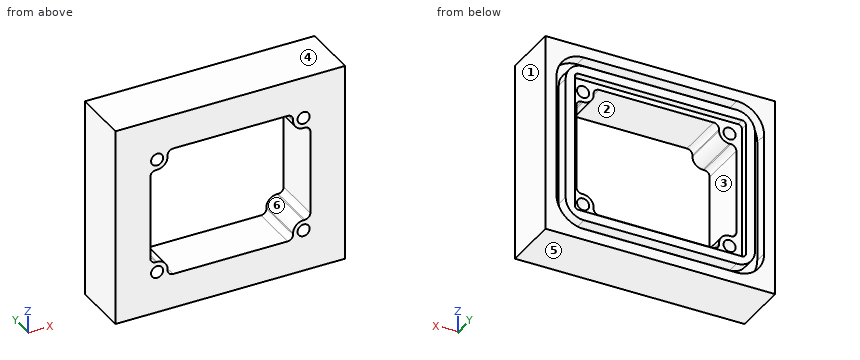
```python
from build123d import *

# Parameters (mm, degrees)
SKETCH1_W           = 62.705
SKETCH1_H           = 54.455
SKETCH1_R           = 1.65288
BOSS_EXTRUDE1_DEPTH = 15.5
SKETCH2_W           = 46.705
SKETCH2_H           = 38.455
CUT_EXTRUDE1_DEPTH  = 2.024
FILLET2_R           = 1.5
SKETCH3_W           = 56.705
SKETCH3_H           = 48.455
SKETCH3_W_2         = 51.705
SKETCH3_H_2         = 43.455
CUT_EXTRUDE2_DEPTH  = 3.5
FILLET3_R           = 1
FILLET4_R           = 5
FILLET5_R           = 7.5


with BuildPart() as part:
    # Sketch1 → Boss-Extrude1 (new body)
    with BuildSketch(Plane(origin=(0, 0, 0), x_dir=(1, 0, 0), z_dir=(0, 1, 0))):
        Rectangle(SKETCH1_W, SKETCH1_H)
        with Locations(Location((-19.995, 15.87, 0), (0, 0, 270))):
            Circle(SKETCH1_R, mode=Mode.SUBTRACT)
        with Locations(Location((19.995, 15.87, 0), (0, 0, 90))):
            Circle(SKETCH1_R, mode=Mode.SUBTRACT)
        with Locations(Location((19.995, -15.87, 0), (0, 0, 270))):
            Circle(SKETCH1_R, mode=Mode.SUBTRACT)
        with Locations(Location((-19.995, -15.87, 0), (0, 0, 90))):
            Circle(SKETCH1_R, mode=Mode.SUBTRACT)
        with BuildLine():
            Line((21.8525, 13.0125), (21.8525, -13.0125))
            Line((21.8525, -13.0125), (19.995, -13.0125))
            ThreePointArc((19.995, -13.0125), (17.974442373, -13.849442373), (17.1375, -15.87))
            Line((17.1375, -15.87), (17.1375, -17.7275))
            Line((17.1375, -17.7275), (-17.1375, -17.7275))
            Line((-17.1375, -17.7275), (-17.1375, -15.87))
            ThreePointArc((-17.1375, -15.87), (-17.974442373, -13.849442373), (-19.995, -13.0125))
            Line((-19.995, -13.0125), (-21.8525, -13.0125))
            Line((-21.8525, -13.0125), (-21.8525, 13.0125))
            Line((-21.8525, 13.0125), (-19.995, 13.0125))
            ThreePointArc((-19.995, 13.0125), (-17.974442373, 13.849442373), (-17.1375, 15.87))
            Line((-17.1375, 15.87), (-17.1375, 17.7275))
            Line((-17.1375, 17.7275), (17.1375, 17.7275))
            Line((17.1375, 17.7275), (17.1375, 15.87))
            ThreePointArc((17.1375, 15.87), (17.974442373, 13.849442373), (19.995, 13.0125))
            Line((19.995, 13.0125), (21.8525, 13.0125))
        make_face(mode=Mode.SUBTRACT)
    extrude(amount=BOSS_EXTRUDE1_DEPTH)

    # Sketch2 → Cut-Extrude1 (cut)
    with BuildSketch(Plane(origin=(0, 15.5, 0), x_dir=(1, 0, 0), z_dir=(0, 1, 0))):
        Rectangle(SKETCH2_W, SKETCH2_H)
    extrude(amount=-CUT_EXTRUDE1_DEPTH, mode=Mode.SUBTRACT)

    # Fillet2
    fillet2_edges = [part.edges().sort_by_distance(p)[0] for p in [
        (21.8525, 6.738, -13.0125),
        (21.8525, 6.738, 13.0125),
        (17.1375, 6.738, 17.7275),
        (-17.1375, 6.738, 17.7275),
        (-21.8525, 6.738, 13.0125),
        (-21.8525, 6.738, -13.0125),
        (-17.1375, 6.738, -17.7275),
        (17.1375, 6.738, -17.7275),
    ]]
    fillet(fillet2_edges, radius=FILLET2_R)

    # Sketch3 → Cut-Extrude2 (cut)
    with BuildSketch(Plane(origin=(0, 15.5, 0), x_dir=(1, 0, 0), z_dir=(0, 1, 0))):
        Rectangle(SKETCH3_W, SKETCH3_H)
        Rectangle(SKETCH3_W_2, SKETCH3_H_2, mode=Mode.SUBTRACT)
    extrude(amount=-CUT_EXTRUDE2_DEPTH, mode=Mode.SUBTRACT)

    # Fillet3
    fillet3_edges = [part.edges().sort_by_distance(p)[0] for p in [
        (-23.3525, 14.488, 19.2275),
        (-23.3525, 14.488, -19.2275),
        (23.3525, 14.488, -19.2275),
        (23.3525, 14.488, 19.2275),
    ]]
    fillet(fillet3_edges, radius=FILLET3_R)

    # Fillet4
    fillet4_edges = [part.edges().sort_by_distance(p)[0] for p in [
        (-25.8525, 13.75, 21.7275),
        (-25.8525, 13.75, -21.7275),
        (25.8525, 13.75, -21.7275),
        (25.8525, 13.75, 21.7275),
    ]]
    fillet(fillet4_edges, radius=FILLET4_R)

    # Fillet5
    fillet5_edges = [part.edges().sort_by_distance(p)[0] for p in [
        (-28.3525, 13.75, 24.2275),
        (-28.3525, 13.75, -24.2275),
        (28.3525, 13.75, -24.2275),
        (28.3525, 13.75, 24.2275),
    ]]
    fillet(fillet5_edges, radius=FILLET5_R)


solid = part.part
```
Verification items for the finished model (mm, model axes). Face numbers are marked on the shaded views. A direction names the side the tool comes from. Coordinates: 2 decimals unless noted, no trailing zeros. Loops run counter-clockwise (first coordinate to the right, second up) from the corner with the lowest first, then second, coordinate; pieces in that order, holes last. Notation, with made-up numbers: (-9, 68.5) - (29, 68.5) arc R17 cw to (29, 77.5) - close; hole circle Ø9 at (23, -16.75). An arc over 180 degrees is marked (long way). Put each result on its own line as item: value.
Item 1: Set-up check for the marked faces 5 and 6: record each of +Z, -Z, +X, -X, +Y, -Y from which the full face is reachable in a straight line by a thin tool's end or side.
Conclusion:
face 5: -Z, +X, -X, +Y, -Y
face 6: +Y, -Y
Item 2: Scan lines: line 1 along X through (y, z) = (4.25, 15.87); line 2 along Z through (x, y) = (-2.5, 3); line 3 along X through (y, z) = (8.5, -1.5). Record each from-to range of solid material in increasing order.
Conclusion:
line 1: x = -31.35 to -21.65, -18.34 to -17.14, 17.14 to 18.34, 21.65 to 31.35
line 2: z = -27.23 to -17.73, 17.73 to 27.23
line 3: x = -31.35 to -21.85, 21.85 to 31.35
Item 3: Section check A-A (x = -9.5). Enter the section's corners in (y, z), then the cut area to 3 significant figures.
Conclusion:
outline: (0, -27.23) - (15.5, -27.23) - (15.5, -24.23) - (12, -24.23) - (12, -21.73) - (15.5, -21.73) - (15.5, -19.23) - (13.48, -19.23) - (13.48, -17.73) - (0, -17.73) - close; (0, 17.73) - (13.48, 17.73) - (13.48, 19.23) - (15.5, 19.23) - (15.5, 21.73) - (12, 21.73) - (12, 24.23) - (15.5, 24.23) - (15.5, 27.23) - (0, 27.23) - close
area: 271 mm2
Item 4: Gauge pin test, flat end, axial feed: pin 1 Ø2.5 at (x, z) = (-19.995, 15.87) entering from -Y. Record the tip position at first contact, or that the pin passes through.
Conclusion:
pin 1: passes through
Item 5: Section check C-C (z = -21). Enter the section's corners in (x, y), then the cut area to 3 significant figures.
Conclusion:
outline: (-31.35, 0) - (31.35, 0) - (31.35, 15.5) - (27.02, 15.5) - (27.02, 12) - (23.45, 12) - (23.45, 15.5) - (-23.45, 15.5) - (-23.45, 12) - (-27.02, 12) - (-27.02, 15.5) - (-31.35, 15.5) - close
area: 947 mm2
Item 6: Draft check along Z on the marked faces 1, 2, 3 and 4. Enter one of: pulls with the +Z half, pulls with the -Z half, needs draft (parallel to the pull), parting line crosses it, or undercut.
Conclusion:
face 1: needs draft
face 2: undercut
face 3: undercut
face 4: pulls with the +Z half
Item 7: Section check B-B (y = 10.5). Give the number of separate pieces and of enclosed holes in the cut face, then the cut area to 3 significant figures.
Conclusion:
separate pieces: 1
enclosed holes: 5
area: 1,920 mm2
